Check sheet for the modelled part. Datum: model origin and axes. Units: mm. A direction names the side the tool comes from. Give positions to 0.01 mm unless a question says otherwise; leave off trailing zeros. Order: outer loops, then holes, each group sorted by start corner. A loop starts at its lowest first (then second) coordinate and runs counter-clockwise, first axis right, second up.
Item 1: Material ranges on line 1 along X through (y, z) = (2.1, -5); line 2 along X through (y, z) = (-3, -20.5); line 3 along Z through (x, y) = (109.5, 2), recorded low to high.
Item 2: Access from +Z, -Z, +X, -X, +Y, -Y to the whole of each face (thin tool, end or side, straight path). Record for faces 1 (the cylindrical face through (113, 1, -1)), 2 (the flat face through (22.544, 2.746, -46.354)), 3 (the cylindrical face through (32.12, -2.46, -19.53)).
Item 3: Release check for a two-part mould opening along Z. For faces 4 (the flat face through (55, 0, -59)), 5 (the cylindrical face through (114, 1, -94)), 6 (the cylindrical face through (88.583, -2.465, -59.241)), 7 (the flat face through (12, 2.5, -52)) record: released by +Z, released by -Z, zero draft, split by the parting line, or undercut.
Item 4: Sectioned sample at D-D on x = 92. Record the boundary of the cut face in (y, z), and give its area (3 significant figures).
Item 5: Sectioned sample at C-C on x = 17.5. Record the boundary of the cut face in (y, z).
Item 6: Gauge pin test, flat end, axial feed: P1, Ø1.4, axis at x = 31.5, z = -21, coming from the -Y side. Record the tip position at first contact, or that the pin passes through.
Item 7: Sectioned sample at A-A on y = -3. Count the separate pieces of the cut face and the enclosed holes in it, and give its area (3 significant figures).
Item 8: Sectioned sample at B-B on z = -83. Record the boundary of the cut face in (x, y).
from build123d import *

# Parameters (mm, degrees)
BOSS_EXTRUDE1_DEPTH     = 3
CUT_EXTRUDE2_DEPTH      = 150.833240638
CUT_EXTRUDE2_DEPTH_BACK = 150.833240638
SKETCH3_R               = 1.6
CUT_EXTRUDE3_DEPTH      = 150.833240638
CUT_EXTRUDE3_DEPTH_BACK = 150.833240638
SKETCH5_W               = 2
SKETCH5_H               = 22.4
SKETCH6_R               = 3.5
SKETCH6_R_2             = 1.45
BOSS_EXTRUDE2_DEPTH     = 5
SKETCH8_R               = 3.25
CUT_EXTRUDE5_DEPTH      = 151.016665741
CUT_EXTRUDE10_START     = -0.5
CUT_EXTRUDE10_DEPTH     = 0.5


# Read off the part's stored shape, not the designer's step: Cut-Extrude10
with BuildPart() as part:
    # Sketch1 → Boss-Extrude1 (new body)
    with BuildSketch(Plane(origin=(0, 0, 0), x_dir=(1, 0, 0), z_dir=(0, 1, 0))):
        with BuildLine():
            Line((5, 0), (110, 0))
            ThreePointArc((110, 0), (113.535533906, 1.464466094), (115, 5))
            Line((115, 5), (115, 91))
            ThreePointArc((115, 91), (113.535533906, 94.535533906), (110, 96))
            Line((110, 96), (5, 96))
            ThreePointArc((5, 96), (1.464466094, 94.535533906), (0, 91))
            Line((0, 91), (0, 5))
            ThreePointArc((0, 5), (1.464466094, 1.464466094), (5, 0))
        make_face()
    extrude(amount=BOSS_EXTRUDE1_DEPTH)

    # Sketch3 → Cut-Extrude2 (cut, two sides: drawn at the far end of the back side and taken through both)
    with BuildSketch(Plane.XZ.offset(-CUT_EXTRUDE2_DEPTH_BACK)):
        with Locations(Location((30.5, -91, 0), (0, 0, 270))):
            Circle(SKETCH3_R)
        with Locations(Location((110, -91, 0), (0, 0, 270))):
            Circle(SKETCH3_R)
        with Locations(Location((110, -5, 0), (0, 0, 270))):
            Circle(SKETCH3_R)
        with Locations(Location((30.5, -5, 0), (0, 0, 270))):
            Circle(SKETCH3_R)
    extrude(amount=CUT_EXTRUDE2_DEPTH + CUT_EXTRUDE2_DEPTH_BACK, mode=Mode.SUBTRACT)

    # Sketch5 → Cut-Extrude3 (cut, two sides: drawn at the far end of the back side and taken through both)
    with BuildSketch(Plane(origin=(0, 3, 0), x_dir=(1, 0, 0), z_dir=(0, 1, 0)).offset(-CUT_EXTRUDE3_DEPTH_BACK)):
        with Locations((112, 36)):
            Rectangle(SKETCH5_W, SKETCH5_H)
    extrude(amount=CUT_EXTRUDE3_DEPTH + CUT_EXTRUDE3_DEPTH_BACK, mode=Mode.SUBTRACT)

    # Sketch6 → Boss-Extrude2 (add)
    # profile 1 of 5: a face of its own
    with BuildSketch(Plane.XZ):
        with Locations(Location((12.34, -37.36, 0), (0, 0, 270))):
            Circle(SKETCH6_R)
        with Locations(Location((12.34, -37.36, 0), (0, 0, 270))):
            Circle(SKETCH6_R_2, mode=Mode.SUBTRACT)
    # profile 2 of 5: a face of its own
    with BuildSketch(Plane.XZ):
        with Locations(Location((31.14, -20.6, 0), (0, 0, 270))):
            Circle(SKETCH6_R)
        with Locations(Location((31.14, -20.6, 0), (0, 0, 270))):
            Circle(SKETCH6_R_2, mode=Mode.SUBTRACT)
    # profile 3 of 5: a face of its own
    with BuildSketch(Plane.XZ):
        with Locations(Location((80, -23, 0), (0, 0, 270))):
            Circle(SKETCH6_R)
        with Locations(Location((80, -23, 0), (0, 0, 270))):
            Circle(SKETCH6_R_2, mode=Mode.SUBTRACT)
    # profile 4 of 5: a face of its own
    with BuildSketch(Plane.XZ):
        with Locations(Location((55, -58.7, 0), (0, 0, 270))):
            Circle(SKETCH6_R)
        with Locations(Location((55, -58.7, 0), (0, 0, 270))):
            Circle(SKETCH6_R_2, mode=Mode.SUBTRACT)
    # profile 5 of 5: a face of its own
    with BuildSketch(Plane.XZ):
        with Locations(Location((92, -60, 0), (0, 0, 270))):
            Circle(SKETCH6_R)
        with Locations(Location((92, -60, 0), (0, 0, 270))):
            Circle(SKETCH6_R_2, mode=Mode.SUBTRACT)
    extrude(amount=BOSS_EXTRUDE2_DEPTH)

    # Sketch8 → Cut-Extrude5 (cut, through all)
    with BuildSketch(Plane(origin=(0, 3, 0), x_dir=(1, 0, 0), z_dir=(0, 1, 0))):
        with Locations(Location((100.830700964, 83.447928687, 0), (0, 0, 270))):
            Circle(SKETCH8_R)
    extrude(amount=-CUT_EXTRUDE5_DEPTH, mode=Mode.SUBTRACT)

    # Cut-Extrude10 outline → Cut-Extrude10 (cut)
    # profile 1 of 5: a face of its own
    with BuildSketch(Plane(origin=(0, 3, 0), x_dir=(1, 0, 0), z_dir=(0, 1, 0)).offset(CUT_EXTRUDE10_START)):
        with BuildLine():
            add(Edge.make_bspline(
                [(33.297546512, 60.762111078), (34.321493225, 61.048834598), (36.18852417, 62.550801835), (39.070738928, 60.462755537), (42.712636812, 60.208352882), (43.144004006, 56.602527257), (46.09833526, 54.669098205), (45.006476912, 51.26118059), (46.336556679, 47.589715296), (42.682432836, 46.184375587), (42.072894551, 42.321191178), (38.279932777, 42.959244425), (35.262379734, 40.642228973), (32.814739239, 43.620013549), (29.131791016, 43.12301619), (28.257625721, 46.713581483), (24.638110416, 48.904686116), (27.648013187, 52.086935615), (25.349884181, 55.492167671), (28.714558965, 57.399923404), (29.840222465, 60.781714479), (32.27004315, 60.474391631), (33.297546512, 60.762111078)],
                knots=[0, 0, 0, 0, 0.047565866, 0.099485372, 0.14962398, 0.198942511, 0.245793773, 0.294983717, 0.351097127, 0.397671231, 0.448622997, 0.49991252, 0.548427096, 0.601372094, 0.646990452, 0.695732934, 0.75340056, 0.801073119, 0.852346593, 0.899993152, 0.952268916, 1, 1, 1, 1], degree=3))
        make_face()
    # profile 2 of 5: a face of its own
    with BuildSketch(Plane(origin=(0, 3, 0), x_dir=(1, 0, 0), z_dir=(0, 1, 0)).offset(CUT_EXTRUDE10_START)):
        with BuildLine():
            add(Edge.make_bspline(
                [(99.964766601, 61.220545167), (100.791800419, 61.220545167), (102.365079498, 60.960449653), (103.919562133, 59.691685536), (104.957768655, 58.295336972), (105.985657449, 56.088458462), (105.896217849, 53.802166915), (105.066743657, 52.572435992)],
                knots=[0, 0, 0, 0, 0.198500718, 0.395419287, 0.481006054, 0.634425351, 1, 1, 1, 1], degree=3))
            Line((99.964766601, 61.220545167), (89.256491407, 61.220545167))
            Line((89.256491407, 61.220545167), (89.256491407, 42.459618206))
            Line((89.256491407, 42.459618206), (101.719296112, 42.459618206))
            add(Edge.make_bspline(
                [(101.719296112, 42.459618206), (103.54789728, 42.555591833), (105.687893164, 44.259558049), (107.07317679, 47.24879867), (106.917803922, 49.989164315), (106.110293292, 51.843021102), (105.066743657, 52.572435992)],
                knots=[0, 0, 0, 0, 0.392551362, 0.572802732, 0.719790987, 1, 1, 1, 1], degree=3))
        make_face()
        with BuildLine():
            Line((100.884956632, 47.819883052), (94.693178468, 47.819883052))
            Line((94.693178468, 47.819883052), (94.693178468, 49.239355876))
            Line((94.693178468, 49.239355876), (100.884956632, 49.239355876))
            ThreePointArc((100.884956632, 49.239355876), (101.594693044, 48.529619464), (100.884956632, 47.819883052))
        make_face(mode=Mode.SUBTRACT)
        with BuildLine():
            Line((94.693178468, 54.49229736), (94.693178468, 55.750824339))
            Line((94.693178468, 55.750824339), (99.591229416, 55.750824339))
            ThreePointArc((99.591229416, 55.750824339), (100.220492906, 55.121560849), (99.591229416, 54.49229736))
            Line((99.591229416, 54.49229736), (94.693178468, 54.49229736))
        make_face(mode=Mode.SUBTRACT)
    # profile 3 of 5: a face of its own
    with BuildSketch(Plane(origin=(0, 3, 0), x_dir=(1, 0, 0), z_dir=(0, 1, 0)).offset(CUT_EXTRUDE10_START)):
        with BuildLine():
            Line((24.604540144, 44.382816286), (20.424423017, 48.381106705))
            ThreePointArc((20.424423017, 48.381106705), (12.555614195, 51.633082316), (20.425070456, 54.883490876))
            Line((20.425070456, 54.883490876), (24.535811062, 58.952326397))
            ThreePointArc((24.535811062, 58.952326397), (6.771833422, 51.583610816), (24.604540144, 44.382816286))
        make_face()
    # profile 4 of 5: a face of its own
    with BuildSketch(Plane(origin=(0, 3, 0), x_dir=(1, 0, 0), z_dir=(0, 1, 0)).offset(CUT_EXTRUDE10_START)):
        Polygon((64.279295174, 47.819883052), (54.324517603, 47.819883052), (54.324517603, 61.220545167), (48.734527121, 61.220545167), (48.734527121, 42.459618206), (64.279295174, 42.459618206), align=None)
    # profile 5 of 5: a face of its own
    with BuildSketch(Plane(origin=(0, 3, 0), x_dir=(1, 0, 0), z_dir=(0, 1, 0)).offset(CUT_EXTRUDE10_START)):
        Polygon((80.447099228, 45.850476979), (82.001118719, 42.459618206), (87.332392702, 42.459618206), (79.844494259, 61.212980487), (73.562845062, 61.212980487), (66.081854559, 42.459618206), (71.643767403, 42.459618206), (72.996430562, 45.850476979), align=None)
        Polygon((76.683077803, 55.362370529), (78.274991903, 51.37543854), (75.09263232, 51.37543854), align=None, mode=Mode.SUBTRACT)
    extrude(amount=CUT_EXTRUDE10_DEPTH, mode=Mode.SUBTRACT)


solid = part.part
Report:
1. line 1: x = 0 to 28.9, 32.1 to 108.4, 111.6 to 115
1. line 2: x = 27.64 to 29.69, 32.59 to 34.64, 77.55 to 82.45
1. line 3: z = -96 to -92.52, -89.48 to -6.52, -3.48 to 0
2. face 1: +Z, +X, +Y, -Y
2. face 2: +Y
2. face 3: -Y
3. face 4: undercut
3. face 5: released by -Z
3. face 6: split by the parting line
3. face 7: undercut
4. outline: (-5, -63.5) - (0, -63.5) - (0, -96) - (3, -96) - (3, -61.22) - (2.5, -61.22) - (2.5, -42.46) - (3, -42.46) - (3, 0) - (0, 0) - (0, -56.5) - (-5, -56.5) - (-5, -58.55) - (0, -58.55) - (0, -61.45) - (-5, -61.45) - close
4. area: 299 mm2
5. outline: (0, -96) - (3, -96) - (3, -62.02) - (2.5, -62.02) - (2.5, -56.23) - (3, -56.23) - (3, -47.04) - (2.5, -47.04) - (2.5, -41.25) - (3, -41.25) - (3, 0) - (0, 0) - close
6. P1: stops at y = 0
7. separate pieces: 5
7. enclosed holes: 5
7. area: 159 mm2
8. outline: (0, 0) - (97.61, 0) - (97.61, 3) - (0, 3) - close; (104.05, 0) - (115, 0) - (115, 3) - (104.05, 3) - close
